Source: three-view drawing plus pictorial views. Frame: mm from the lowest corner of the part. Give positions to 0.01 mm unless a question says otherwise; leave off trailing zeros. Loops run counter-clockwise (first coordinate to the right, second up) from the corner with the lowest first, then second, coordinate; pieces in that order, holes last. Notation, with made-up numbers: (-37, -2) -> (0, -2) arc R17 ccw to (0, 27) -> close; hole circle Ø8 at (-33, 5.5). An arc over 180 degrees is marked (long way). Answer in a Markdown table with one row per item. Add a question column.
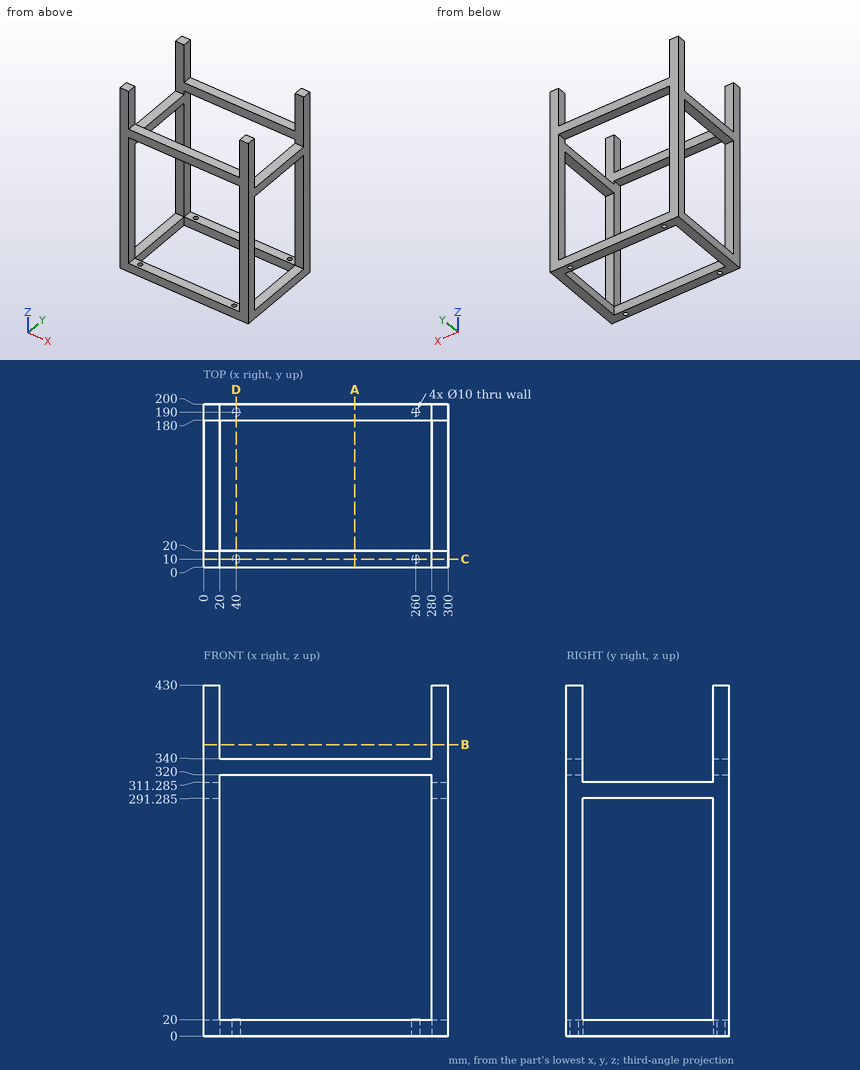
(1) Pin query (flat end, axial travel): pin 1 Ø16 at (x, y) = (289.5, 108) entering from +Z (3 decimals); pin 2 Ø10 at (x, y) = (193.5, 6.5) entering from +Z; pin 3 Ø10 at (x, y) = (15, 89.5) entering from -Z. Return the tip coordinate at first contact, or that it passes through.
(2) Cut plane C-C on y = 10. Return the cut outline in (x, z), then the cut area to 3 significant figures.
(3) Cut plane D-D on x = 40. Return the cut outline in (y, z).
(4) Cut plane A-A on x = 185.5. Return the cut outline in (y, z).
(5) Material intervals for line 1 along Y through (x, z) = (260, 14); line 2 along X through (y, z) = (190, 11); line 3 along X through (y, z) = (179, 300.5), sorted ascending. Write a range as from..to.
(6) Cut plane B-B on z = 357. Return the cut outline in (x, y).
Answer list:
| question | item | result |
|---|---|---|
| 1 | pin 1 | stops at z = 311.285 |
| 1 | pin 2 | stops at z = 340 |
| 1 | pin 3 | stops at z = 0 |
| 2 | outline | (0, 0) -> (35, 0) -> (35, 20) -> (20, 20) -> (20, 320) -> (280, 320) -> (280, 20) -> (265, 20) -> (265, 0) -> (300, 0) -> (300, 430) -> (280, 430) -> (280, 340) -> (20, 340) -> (20, 430) -> (0, 430) -> close; (45, 0) -> (255, 0) -> (255, 20) -> (45, 20) -> close |
| 2 | area | 27,200 mm² |
| 3 | outline | (0, 0) -> (5, 0) -> (5, 20) -> (0, 20) -> close; (0, 320) -> (20, 320) -> (20, 340) -> (0, 340) -> close; (15, 0) -> (20, 0) -> (20, 20) -> (15, 20) -> close; (180, 0) -> (185, 0) -> (185, 20) -> (180, 20) -> close; (180, 320) -> (200, 320) -> (200, 340) -> (180, 340) -> close; (195, 0) -> (200, 0) -> (200, 20) -> (195, 20) -> close |
| 4 | outline | (0, 0) -> (20, 0) -> (20, 20) -> (0, 20) -> close; (0, 320) -> (20, 320) -> (20, 340) -> (0, 340) -> close; (180, 0) -> (200, 0) -> (200, 20) -> (180, 20) -> close; (180, 320) -> (200, 320) -> (200, 340) -> (180, 340) -> close |
| 5 | line 1 | y = 0..5, 15..20, 180..185, 195..200 |
| 5 | line 2 | x = 0..35, 45..255, 265..300 |
| 5 | line 3 | x = 0..20, 280..300 |
| 6 | outline | (0, 0) -> (20, 0) -> (20, 20) -> (0, 20) -> close; (0, 180) -> (20, 180) -> (20, 200) -> (0, 200) -> close; (280, 0) -> (300, 0) -> (300, 20) -> (280, 20) -> close; (280, 180) -> (300, 180) -> (300, 200) -> (280, 200) -> close |
